```python
from build123d import *

# Parameters (mm, degrees)
SKETCH1_R           = 7.5
SKETCH1_R_2         = 4.5
BOSS_EXTRUDE1_DEPTH = 12.7


with BuildPart() as part:
    # Sketch1 → Boss-Extrude1 (new body)
    with BuildSketch(Plane.XY):
        Polygon((46.5, -25.264079911), (40.577892741, -37.964079911), (15.177892741, -37.964079911), (9.255785483, -25.264079911), (-9.255785483, -25.264079911), (-15.177892741, -37.964079911), (-40.577892741, -37.964079911), (-46.5, -25.264079911), (-63.5, -25.264079911), (-63.5, 38.235920089), (63.5, 38.235920089), (63.5, -25.264079911), align=None)
        Circle(SKETCH1_R, mode=Mode.SUBTRACT)
        with Locations((31.75, 12.835920089)):
            Circle(SKETCH1_R_2, mode=Mode.SUBTRACT)
        with Locations((-31.75, 12.835920089)):
            Circle(SKETCH1_R_2, mode=Mode.SUBTRACT)
    extrude(amount=BOSS_EXTRUDE1_DEPTH)


solid = part.part
```
For this review, take the finished solid that the model builds, in its own axes (mm). A direction names the side the tool comes from. Give positions to 0.01 mm unless a question says otherwise; leave off trailing zeros. Order: outer loops, then holes, each group sorted by start corner. A loop starts at its lowest first (then second) coordinate and runs counter-clockwise, first axis right, second up.
1) Take a section at C-C (y = 15). Give the boundary of the cut face in (x, z), then the cut area to 3 significant figures.
2) Insertion check: pin 1 (6.5 mm diameter, centred on x = 58.5, z = 4.5, fed in from -Y). The pin has a flat end and moves straight along its axis. Give the tip position at first contact, or say it passes through.
3) The part is to be moulded in two halves that separate along X. For faces 1 (the face through (-63.5, 6, 6)), 2 (the face through (1, 9, 0)), 3 (the face through (0, -25.264, 6)), say which applies: released by +X, released by -X, zero draft, split by the parting line, or undercut.
4) Take a section at B-B (x = 0). Give the boundary of the cut face in (y, z).
5) For faces 4 (the face through (55, -25.264, 6)), 5 (the face through (-7.493, 0.33, 6.261)), 6 (the face through (-28, -37.964, 6)), 7 (the face through (-55, -25.264, 6)), 8 (the face through (12.258, -31.703, 6.261)), list the 3-axis set-ups (+Z, -Z, +X, -X, +Y, -Y) from which the entire face can be reached by the end or side of a thin tool; tool diameter is ignored.
6) Take a section at D-D (z = 11.5). Give the boundary of the cut face in (x, y).
7) Take a section at A-A (y = 0). Give the boundary of the cut face in (x, z).
8) Wall thickness on line 1 (Y direction, x = 31.75, z = 4.75); line 2 (Y direction, x = 0, z = 5.5); line 3 (X direction, y = -25.5, z = 8.25): over which ranges is each line inside the solid? List them lowest first.
Derived:
1. outline: (-63.5, 0) - (-35.7, 0) - (-35.7, 12.7) - (-63.5, 12.7) - close; (-27.8, 0) - (27.8, 0) - (27.8, 12.7) - (-27.8, 12.7) - close; (35.7, 0) - (63.5, 0) - (63.5, 12.7) - (35.7, 12.7) - close
1. area: 1,410 mm2
2. pin 1: stops at y = -25.26
3. face 1: released by -X
3. face 2: zero draft
3. face 3: undercut
4. outline: (-25.26, 0) - (-7.5, 0) - (-7.5, 12.7) - (-25.26, 12.7) - close; (7.5, 0) - (38.24, 0) - (38.24, 12.7) - (7.5, 12.7) - close
5. face 4: +Z, -Z, +X, -Y
5. face 5: +Z, -Z
5. face 6: +Z, -Z, +X, -X, -Y
5. face 7: +Z, -Z, -X, -Y
5. face 8: +Z, -Z, -Y
6. outline: (-63.5, -25.26) - (-46.5, -25.26) - (-40.58, -37.96) - (-15.18, -37.96) - (-9.26, -25.26) - (9.26, -25.26) - (15.18, -37.96) - (40.58, -37.96) - (46.5, -25.26) - (63.5, -25.26) - (63.5, 38.24) - (-63.5, 38.24) - close; hole circle Ø9 at (-31.75, 12.84); hole circle Ø15 at (0, 0); hole circle Ø9 at (31.75, 12.84)
7. outline: (-63.5, 0) - (-7.5, 0) - (-7.5, 12.7) - (-63.5, 12.7) - close; (7.5, 0) - (63.5, 0) - (63.5, 12.7) - (7.5, 12.7) - close
8. line 1: y = -37.96 to 8.34, 17.34 to 38.24
8. line 2: y = -25.26 to -7.5, 7.5 to 38.24
8. line 3: x = -46.39 to -9.37, 9.37 to 46.39
